Check sheet for the drawn part. Datum: minimum x, y, z corner. Units: mm. A direction names the side the tool comes from. Coordinates: 2 decimals unless noted, no trailing zeros. Order: outer loops, then holes, each group sorted by start corner. A loop starts at its lowest first (then second) coordinate and runs counter-clockwise, first axis right, second up. Notation, with made-up numbers: (33.5, -23) - (71.5, -23) arc R32 ccw to (71.5, 13) - close; hole circle Ø8 at (50.25, 30.25). An arc over 180 degrees is marked (long way). Answer as CSV lines item,"result". Start each with the question number.
1. Section check C-C (z = 32). Record the cut outline in (x, y), and give its area (3 significant figures).
2. Section check B-B (x = 40). Record the cut outline in (y, z), and give its area (3 significant figures).
3. Set-up check for the marked faces 1, 2 and 3: record each of +Z, -Z, +X, -X, +Y, -Y from which the full face is reachable in a straight line by a thin tool's end or side.
4. Mould release check, pull along X, two halves, no side actions. Record for the marked faces 4, 5 and 6: pulls with the +X half, pulls with the -X half, needs draft (parallel to the pull), parting line crosses it, or undercut.
5. Go/stop test with flat-tipped pins: pin 1 (8 mm diameter, centred on x = 47, z = 65.5, fed in from +Y); pin 2 (4 mm diameter, centred on x = 39.5, z = 41.5, fed in from +Y); pin 3 (6 mm diameter, centred on y = 138, z = 42.5, fed in from -X); pin 4 (6.5 mm diameter, centred on y = 145, z = 40, fed in from -X). Record where each tip stops, or that it passes through.
6. Section check D-D (y = 18). Record the cut outline in (x, z).
7. Material ranges on L1, parallel to Y at x = 47, z = 40; L2, parallel to Z at x = 32.85, y = 145; L3, parallel to Z at x = 37.5, y = 129.5, recorded low to high. Write a range as [from, to].
8. Section check A-A (z = 40). Record the cut outline in (x, y), and give its area (3 significant figures).
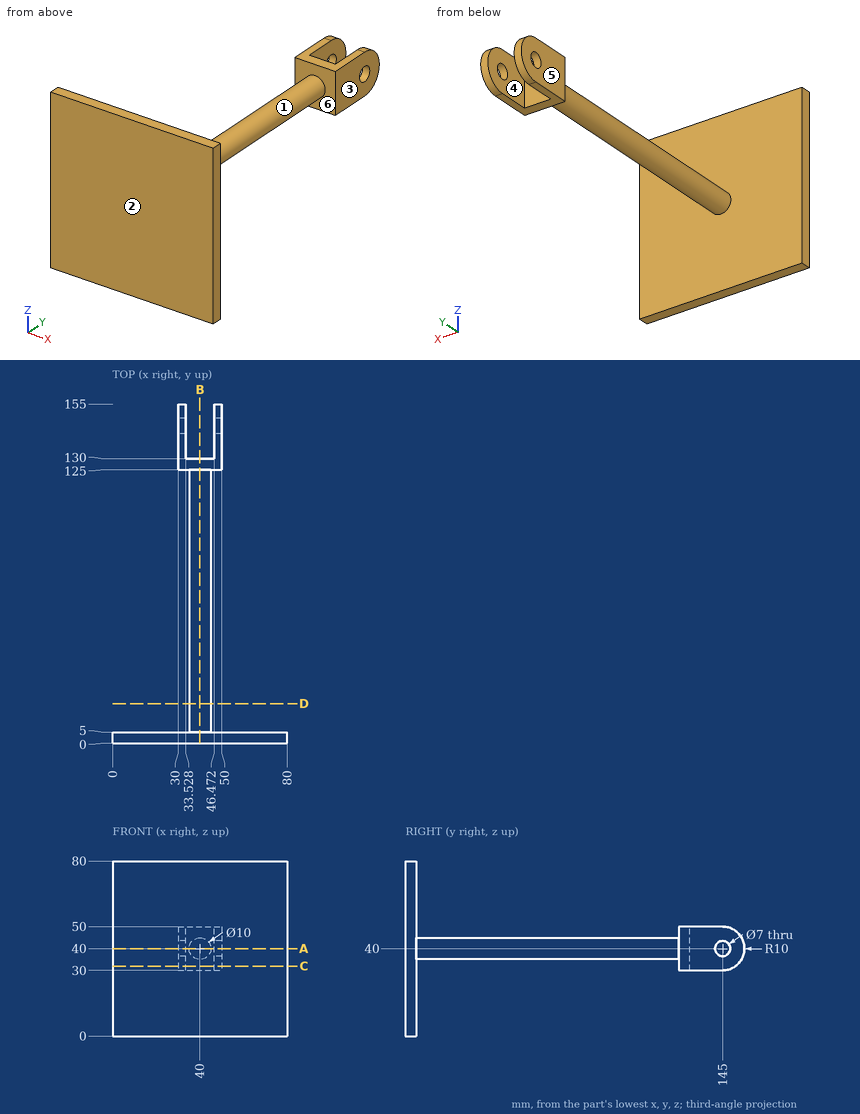
Evaluation:
1,outline,"(0, 0) - (80, 0) - (80, 5) - (0, 5) - close; (30, 125) - (50, 125) - (50, 151) - (46.47, 151) - (46.47, 130) - (33.53, 130) - (33.53, 151) - (30, 151) - close"
1,area,"648 mm²"
2,outline,"(0, 0) - (5, 0) - (5, 35) - (125, 35) - (125, 30) - (130, 30) - (130, 50) - (125, 50) - (125, 45) - (5, 45) - (5, 80) - (0, 80) - close"
2,area,"1,700 mm²"
3,face 1,"none"
3,face 2,"+Z, -Z, +X, -X, -Y"
3,face 3,"+Z, -Z, +X, +Y"
4,face 4,"undercut"
4,face 5,"pulls with the -X half"
4,face 6,"needs draft"
5,pin 1,"stops at y = 5"
5,pin 2,"stops at y = 130"
5,pin 3,"stops at x = 30"
5,pin 4,"passes through"
6,outline,"circle Ø10 at (40, 40)"
7,L1,"y = [0, 5], [125, 141.5], [148.5, 155]"
7,L2,"z = [30, 36.5], [43.5, 50]"
7,L3,"z = [30, 50]"
8,outline,"(0, 0) - (80, 0) - (80, 5) - (45, 5) - (45, 125) - (50, 125) - (50, 141.5) - (46.47, 141.5) - (46.47, 130) - (33.53, 130) - (33.53, 141.5) - (30, 141.5) - (30, 125) - (35, 125) - (35, 5) - (0, 5) - close; (30, 148.5) - (33.53, 148.5) - (33.53, 155) - (30, 155) - close; (46.47, 148.5) - (50, 148.5) - (50, 155) - (46.47, 155) - close"
8,area,"1,830 mm²"
